Source: CAD feature listing. Evaluate the final solid. Frame: model axes, mm. Face numbers are marked on the shaded views. A direction names the side the tool comes from. Round coordinates to 2 decimals unless told otherwise and drop trailing zeros. Order: outer loops, then holes, each group sorted by start corner. A loop starts at its lowest first (then second) coordinate and runs counter-clockwise, first axis right, second up. Notation, with made-up numbers: (-34, -38.5) - (3, -38.5) arc R24 ccw to (3, -1.5) - close; hole circle Ø2 at (-32, 1.5). An arc over 180 degrees is marked (long way). Return JSON: item names as keys, results as strings. Group by question number.
1) Section A-A, the plane z = 23. Return loops of the section in (x, y).
2) Section B-B, the plane x = -14.5. Return loops of the section in (y, z).
3) Section D-D, the plane z = -6.5. Return loops of the section in (x, y), plus the area to 3 significant figures.
4) Mould query, pull axis Y, two halves, no side actions, for the marked faces 4, 5 and 6. Classes: pulls with the +Y half, pulls with the -Y half, needs draft (parallel to the pull), parting line crosses it, or undercut.
5) Contact query for flat-ended pins moving along their axis: P1, Ø12.5, axis at y = -8, z = 13, coming from the +X side; P2, Ø1.5, axis at y = -16.5, z = 4, coming from the -X side; P3, Ø6, axis at y = -12.5, z = -4.5, coming from the -X side. Output: stop coordinate, or through.
6) Section C-C, the plane y = -10.5. Return loops of the section in (x, z).
7) Ray query, line 1 (Y direction, x = -23.5, z = 26); line 2 (X direction, y = -10.5, z = -10); line 3 (Y direction, x = 9, z = -6). Return the intervals inside material, ascending. Write a range as from..to.
8) Access query for the marked faces 1, 2 and 3. Directions: +Z, -Z, +X, -X, +Y, -Y. A direction counts if a zero-diameter tool reaches every point of the face in a straight line with its end or side. Return the directions, or none.
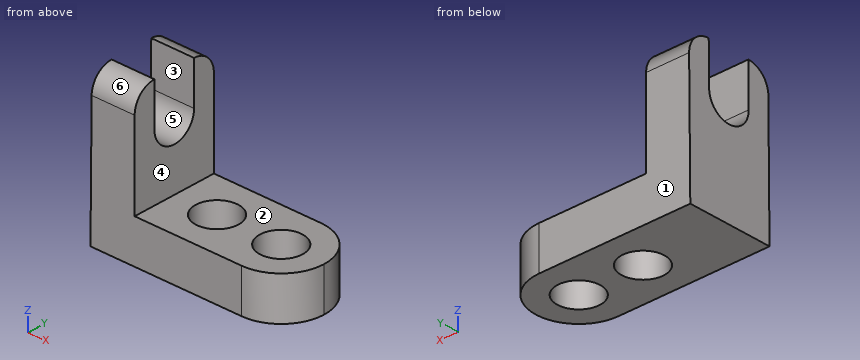
```python
from build123d import *

# Parameters (mm, degrees)
F1_DEPTH = 25.4
F2_R     = 6.35
F3_DEPTH = 25.4
F5_DEPTH = 25.4
F7_DEPTH = 25.4


with BuildPart() as f1:
    # F0 (on Front) → F1 (new body)
    with BuildSketch(Plane.XZ):
        Polygon((-22.412052, 32.592865), (-35.112052, 32.592865), (-35.519832, -11.855265), (22.037948, -11.855265), (22.037948, 0.844735), (-22.412052, 0.844735), align=None)
    extrude(amount=F1_DEPTH)

    # F2 (on face) → F3 (cut)
    with BuildSketch(Plane.XY.offset(0.844735)):
        with Locations((-9.712052, -12.7)):
            Circle(F2_R)
        with Locations((9.337948, -12.7)):
            Circle(F2_R)
        with BuildLine():
            Line((22.037948, 0), (9.337948, 0))
            ThreePointArc((9.337948, 0), (18.318204, -3.719744), (22.037948, -12.7))
            Line((22.037948, -12.7), (22.037948, 0))
        make_face()
        with BuildLine():
            Line((22.037948, -25.4), (22.037948, -12.7))
            ThreePointArc((22.037948, -12.7), (18.318204, -21.680256), (9.337948, -25.4))
            Line((9.337948, -25.4), (22.037948, -25.4))
        make_face()
    extrude(amount=-F3_DEPTH, mode=Mode.SUBTRACT)

    # F4 (on face) → F5 (cut)
    with BuildSketch(Plane.YZ.offset(-22.412052)):
        with BuildLine():
            ThreePointArc((-25.4, 26.242865), (-23.540128, 30.732993), (-19.05, 32.592865))
            Line((-19.05, 32.592865), (-25.4, 32.592865))
            Line((-25.4, 32.592865), (-25.4, 26.242865))
        make_face()
        with BuildLine():
            Line((0, 32.592865), (-6.35, 32.592865))
            ThreePointArc((-6.35, 32.592865), (-1.859872, 30.732993), (0, 26.242865))
            Line((0, 26.242865), (0, 32.592865))
        make_face()
    extrude(amount=-F5_DEPTH, mode=Mode.SUBTRACT)

    # F6 (on face) → F7 (cut)
    with BuildSketch(Plane.YZ.offset(-22.412052)):
        with BuildLine():
            ThreePointArc((-19.05, 19.894735), (-12.7, 26.244735), (-6.35, 19.894735))
            Line((-6.35, 19.894735), (-6.35, 32.592865))
            Line((-6.35, 32.592865), (-19.05, 32.592865))
            Line((-19.05, 32.592865), (-19.05, 19.894735))
        make_face()
        with BuildLine():
            ThreePointArc((-19.05, 19.894735), (-12.7, 13.544735), (-6.35, 19.894735))
            ThreePointArc((-6.35, 19.894735), (-12.7, 26.244735), (-19.05, 19.894735))
        make_face()
    extrude(amount=-F7_DEPTH, mode=Mode.SUBTRACT)


solid = f1.part
```
Geometry check:
{
 "1": {"outline": "(-35.2, -25.4) - (-22.41, -25.4) - (-22.41, -19.05) - (-35.2, -19.05) - close; (-35.2, -6.35) - (-22.41, -6.35) - (-22.41, 0) - (-35.2, 0) - close"},
 "2": {"outline": "(-25.4, -11.86) - (-16.87, -11.86) - (-16.87, 0.84) - (-25.4, 0.84) - close; (-8.53, -11.86) - (0, -11.86) - (0, 0.84) - (-8.53, 0.84) - close"},
 "3": {"outline": "(-35.47, -25.4) - (9.34, -25.4) arc R12.7 ccw to (9.34, 0) - (-35.47, 0) - close; hole circle Ø12.7 at (-9.71, -12.7); hole circle Ø12.7 at (9.34, -12.7)", "area": "1,140 mm2"},
 "4": {"face 4": "needs draft", "face 5": "undercut", "face 6": "pulls with the -Y half"},
 "5": {"P1": "x = -22.41", "P2": "x = -35.38", "P3": "x = -35.48"},
 "6": {"outline": "(-35.52, -11.86) - (-15.67, -11.86) - (-15.67, 0.84) - (-22.41, 0.84) - (-22.41, 13.94) - (-35.28, 13.94) - close; (-3.76, -11.86) - (3.38, -11.86) - (3.38, 0.84) - (-3.76, 0.84) - close; (15.29, -11.86) - (21.85, -11.86) - (21.85, 0.84) - (15.29, 0.84) - close"},
 "7": {"line 1": "-25.4..-19.05, -6.35..0", "line 2": "-35.5..-15.67, -3.76..3.38, 15.29..21.85", "line 3": "-25.4..-19.04, -6.36..0"},
 "8": {"face 1": "+Z, -Z, +X, -X, +Y", "face 2": "+Z, +X, +Y, -Y", "face 3": "+Z, +X, -X"}
}
